from build123d import *

# Parameters (mm, degrees)
F0_W     = 36
F0_H     = 22
F0_R     = 1.6
F0_R_2   = 0.75
F0_W_2   = 24
F0_H_2   = 13
F1_DEPTH = 4
F2_SIZE  = 2
F3_SIZE  = 0.5


with BuildPart() as f1:
    # F0 (on Top) → F1 (new body)
    with BuildSketch(Plane.XY):
        with Locations((12, 5)):
            Rectangle(F0_W, F0_H)
        with Locations((0, -3)):
            Circle(F0_R, mode=Mode.SUBTRACT)
        with Locations((10, -3)):
            Circle(F0_R, mode=Mode.SUBTRACT)
        with Locations((-3, 6.5)):
            Circle(F0_R_2, mode=Mode.SUBTRACT)
        with Locations((12, 6.5)):
            Rectangle(F0_W_2, F0_H_2, mode=Mode.SUBTRACT)
        with Locations((27, 6.5)):
            Circle(F0_R_2, mode=Mode.SUBTRACT)
    extrude(amount=F1_DEPTH)

    # F2
    f2_edges = [f1.edges().sort_by_distance(p)[0] for p in [
        (-6, -6, 2),
        (30, -6, 2),
        (30, 16, 2),
        (-6, 16, 2),
    ]]
    chamfer(f2_edges, length=F2_SIZE)

    # F3
    f3_edges = [f1.edges().sort_by_distance(p)[0] for p in [
        (-6, 5, 0),
        (-5, 15, 0),
        (-5, -5, 0),
        (12, 16, 0),
        (12, -6, 0),
        (29, 15, 0),
        (29, -5, 0),
        (30, 5, 0),
        (-1.6, -3, 0),
        (8.4, -3, 0),
        (-3.75, 6.5, 0),
        (12, 0, 0),
        (0, 6.5, 0),
        (12, 13, 0),
        (24, 6.5, 0),
        (26.25, 6.5, 0),
        (-6, 5, 4),
        (-5, 15, 4),
        (-5, -5, 4),
        (12, 16, 4),
        (12, -6, 4),
        (29, 15, 4),
        (29, -5, 4),
        (30, 5, 4),
        (-1.6, -3, 4),
        (8.4, -3, 4),
        (-3.75, 6.5, 4),
        (12, 0, 4),
        (0, 6.5, 4),
        (12, 13, 4),
        (24, 6.5, 4),
        (26.25, 6.5, 4),
    ]]
    chamfer(f3_edges, length=F3_SIZE)


solid = f1.part
Input: part model. Units: mm. Frame: model coordinates. A direction names the side the tool comes from. Give positions to 0.01 mm unless a question says otherwise; leave off trailing zeros. Order: outer loops, then holes, each group sorted by start corner. A loop starts at its lowest first (then second) coordinate and runs counter-clockwise, first axis right, second up. Notation, with made-up numbers: (-9.5, 82) -> (-0.5, 82) arc R17 ccw to (-0.5, 97) -> close; hole circle Ø6 at (9, -5). An arc over 180 degrees is marked (long way). Use one line per item in the form item = value.
1) First-contact query: pin 1 Ø1.9 at (x, y) = (0, -3) entering from -Z. Flat tip, straight axial feed; report the tip coordinate or a pass-through.
Response values:
pin_1 = through
2) Section A-A, the plane x = -3. Return loops of the section in (y, z).
Response values:
outline = (-6, 0.5) -> (-5.5, 0) -> (5.25, 0) -> (5.75, 0.5) -> (5.75, 3.5) -> (5.25, 4) -> (-5.5, 4) -> (-6, 3.5) -> close; (7.25, 0.5) -> (7.75, 0) -> (15.5, 0) -> (16, 0.5) -> (16, 3.5) -> (15.5, 4) -> (7.75, 4) -> (7.25, 3.5) -> close
3) Section B-B, the plane y = 6.5. Count the separate pieces of the cut face and the enclosed holes in it, and give its area (3 significant figures).
Response values:
separate_pieces = 4
enclosed_holes = 0
area = 34.0 mm^2
4) Section C-C, the plane x = 10. Return loops of the section in (y, z), and give its area (3 significant figures).
Response values:
outline = (-6, 0.5) -> (-5.5, 0) -> (-5.1, 0) -> (-4.6, 0.5) -> (-4.6, 3.5) -> (-5.1, 4) -> (-5.5, 4) -> (-6, 3.5) -> close; (-1.4, 0.5) -> (-0.9, 0) -> (-0.5, 0) -> (0, 0.5) -> (0, 3.5) -> (-0.5, 4) -> (-0.9, 4) -> (-1.4, 3.5) -> close; (13, 0.5) -> (13.5, 0) -> (15.5, 0) -> (16, 0.5) -> (16, 3.5) -> (15.5, 4) -> (13.5, 4) -> (13, 3.5) -> close
area = 21.7 mm^2
5) Line query: probe 1 along Y at (x, z) = (10, 1.7); probe 2 along Y at (x, z) = (27, 1.3); probe 3 along Y at (x, z) = (6, 2.45). Output: solid intervals per line, ascending.
Response values:
probe_1 = -6 to -4.6, -1.4 to 0, 13 to 16
probe_2 = -6 to 5.75, 7.25 to 16
probe_3 = -6 to 0, 13 to 16
6) Section D-D, the plane z = 1.8. Return loops of the section in (x, y), and give its area (3 significant figures).
Response values:
outline = (-6, -4) -> (-4, -6) -> (28, -6) -> (30, -4) -> (30, 14) -> (28, 16) -> (-4, 16) -> (-6, 14) -> close; hole circle Ø1.5 at (-3, 6.5); hole circle Ø3.2 at (0, -3); hole (0, 0) -> (24, 0) -> (24, 13) -> (0, 13) -> close; hole circle Ø3.2 at (10, -3); hole circle Ø1.5 at (27, 6.5)
area = 452 mm^2
7) Reachability of faces 5 (the flat face through (12, 0, 2)), 6 (the flat face through (16, -2, 4)) from +Z, -Z, +X, -X, +Y, -Y: full face, straight path, thin tool, end or side. Return the list, or none.
Response values:
face_5 = +Z, -Z
face_6 = +Z, +X, -X, +Y, -Y
8) Mould query, pull axis X, two halves, no side actions, for faces 1 (the flat face through (29, 15, 2)), 2 (the flat face through (-5, 15, 2)), 3 (the flat face through (12, -6, 2)), 4 (the flat face through (24, 6, 2)). Classes: pulls with the +X half, pulls with the -X half, needs draft (parallel to the pull), parting line crosses it, or undercut.
Response values:
face_1 = pulls with the +X half
face_2 = pulls with the -X half
face_3 = needs draft
face_4 = undercut
